Print and shaded views of the part. All mm, measured from the part's lowest x, y and z. Give positions to 0.01 mm unless a question says otherwise; leave off trailing zeros. Write each loop counter-clockwise with the first axis right and the second up, starting at its lowest first coordinate (ties: lowest second). Pieces come first, ordered by that corner, then holes. Notation, with made-up numbers: (18.25, -18.75) - (69.25, -18.75) arc R12 ccw to (69.25, -7.75) - close; hole circle Ø7 at (77, 36.25). An arc over 180 degrees is marked (long way). Use one line per item in the form item = value. Start each with the question number.
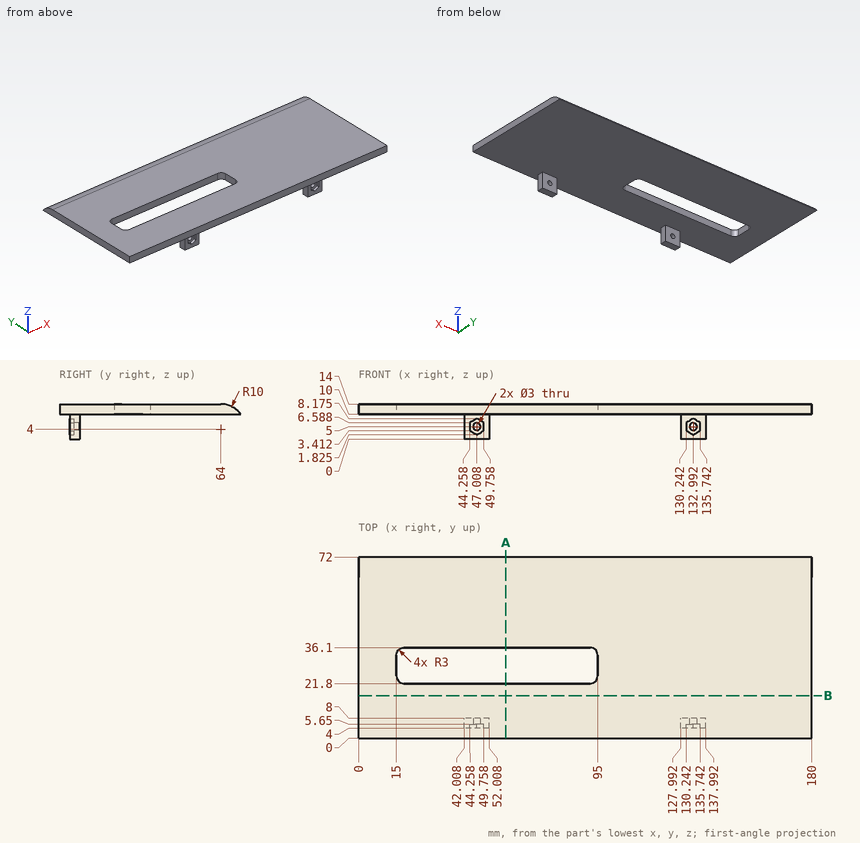
(1) Cut at B-B, the plane y = 17. Give the cut face in (x, z).
(2) Pin check, flat tips, straight feed: pin 1 Ø0.8 at (y, z) = (4.5, 6) entering from +X; pin 2 Ø3 at (x, y) = (93, 64.5) entering from -Z; pin 3 Ø1.2 at (x, z) = (43.5, 12) entering from -Y; pin 4 Ø1.3 at (y, z) = (4.5, 4.5) entering from -X. Stop position of each tip, or through.
(3) Wall check: line 1 (X direction, y = 25, z = 10.75); line 2 (Z direction, x = 118.5, y = 55); line 3 (X direction, y = 5, z = 2.75) (1 decimal). Give the ranges that are in metal, low to high. Write a range as from..to.
(4) Cut at A-A, the plane x = 58.5. Give the cut face in (y, z), then the cut area to 3 significant figures.
Solution:
q1.outline = (0, 10) - (180, 10) - (180, 14) - (0, 14) - close
q2.pin_1 = 137.99
q2.pin_2 = 10
q2.pin_3 = 0
q2.pin_4 = 42.01
q3.line_1 = 0..15, 95..180
q3.line_2 = 10..14
q3.line_3 = 42..45.4, 48.6..52, 128..131.4, 134.6..138
q4.outline = (0, 10) - (21.8, 10) - (21.8, 14) - (0, 14) - close; (36.1, 10) - (72, 10) arc R10 ccw to (64, 14) - (36.1, 14) - close
q4.area = 221 mm2
